The model under review builds one solid part; all positions refer to its coordinate system, in mm. A direction names the side the tool comes from. Coordinates: 2 decimals unless noted, no trailing zeros. Loops run counter-clockwise (first coordinate to the right, second up) from the corner with the lowest first, then second, coordinate; pieces in that order, holes last. Notation, with made-up numbers: M 42.25,77.25 L 59.25,77.25 A17 ccw 59.25,106.25 Z; hole C -4,35.5 d11. An arc over 180 degrees is marked long. Use one line per item in the form item = value.
```python
from build123d import *

# Parameters (mm, degrees)
F2_W = 0.2
F2_H = 0.2


with BuildPart() as f1:
    # F0 (on Right) → F1 (revolve)
    with BuildSketch(Plane.YZ):
        Polygon((-1.5, 0.5), (-1.5, 0), (9.2, 0), (9.2, 0.5), (7.7, 0.5), (7.7, 1.2), (6.2, 1.2), (6.2, 0.5), (3, 0.5), (3, 1.4), (0, 1.4), (0, 0.5), align=None)
    revolve(axis=Axis((0, 3.85, 0), (0, -1, 0)))

    # F2 (on Right) → F3 (revolve, cut)
    with BuildSketch(Plane.YZ):
        with Locations((0.1, 1.3)):
            Rectangle(F2_W, F2_H)
        with Locations((2.9, 1.3)):
            Rectangle(F2_W, F2_H)
    revolve(axis=Axis((0, 1.5, 0), (0, 1, 0)), mode=Mode.SUBTRACT)

    # F4 (on Right) → F5 (revolve)
    with BuildSketch(Plane.YZ):
        Polygon((6.3, 1.2), (6.7, 1.2), (7.6, 1.2), (7.6, 1.4), (6.3, 1.4), align=None)
    revolve(axis=Axis((0, 6.95, 0), (0, 1, 0)))


solid = f1.part
```
1. Add section D-D (y = 8). State the section outline as (x, z) points.
Response values:
outline = C 0,0 d1
2. Add section B-B (x = -0.65). State the section outline as (y, z) points, then the cut area to 3 significant figures.
Response values:
outline = M 0,-1.01 L 0.2,-1.01 L 0.2,-1.24 L 2.8,-1.24 L 2.8,-1.01 L 3,-1.01 L 3,1.01 L 2.8,1.01 L 2.8,1.24 L 0.2,1.24 L 0.2,1.01 L 0,1.01 Z; M 6.2,-1.01 L 6.3,-1.01 L 6.3,-1.24 L 7.6,-1.24 L 7.6,-1.01 L 7.7,-1.01 L 7.7,1.01 L 7.6,1.01 L 7.6,1.24 L 6.3,1.24 L 6.3,1.01 L 6.2,1.01 Z
area = 10.9 mm^2
3. The part is to be moulded in two halves that separate along Y. For faces 4 (the face through (0.488, 8.439, -0.108)), 5 (the face through (1, 3, 0)), 6 (the face through (1, 7.7, 0)), 7 (the face through (0, -1.5, 0)), say which applies: pulls with the +Y half, pulls with the -Y half, needs draft (parallel to the pull), parting line crosses it, or undercut.
Response values:
face_4 = needs draft
face_5 = undercut
face_6 = pulls with the +Y half
face_7 = pulls with the -Y half
4. Add section A-A (z = 0.65). State the section outline as (x, y) points, then the cut area to 3 significant figures.
Response values:
outline = M -1.24,0.2 L -1.01,0.2 L -1.01,0 L 1.01,0 L 1.01,0.2 L 1.24,0.2 L 1.24,2.8 L 1.01,2.8 L 1.01,3 L -1.01,3 L -1.01,2.8 L -1.24,2.8 Z; M -1.24,6.3 L -1.01,6.3 L -1.01,6.2 L 1.01,6.2 L 1.01,6.3 L 1.24,6.3 L 1.24,7.6 L 1.01,7.6 L 1.01,7.7 L -1.01,7.7 L -1.01,7.6 L -1.24,7.6 Z
area = 10.9 mm^2
5. Wall thickness on line 1 along Y through (x, z) = (-0.95, -0.65); line 2 along Y through (x, z) = (-1.1, 0.8); line 3 along X through (y, z) = (5, -0.15): over which ranges is each line inside the solid? List them lowest first. Write a range as from..to.
Response values:
line_1 = 0..3, 6.2..7.7
line_2 = 0.2..2.8, 6.3..7.6
line_3 = -0.48..0.48
6. Machinability: for faces 1 (the face through (1, 6.2, 0)), 2 (the face through (0.06, 6.94, -1.4)), 3 (the face through (1, 0, 0)), which of the approach directions +Z, -Z, +X, -X, +Y, -Y give a long, thin tool a straight path to every point of the face, cutting with its end or side? Answer none if there is none.
Response values:
face_1 = none
face_2 = +Y, -Y
face_3 = -Y
7. Add section C-C (y = 1). State the section outline as (x, z) points.
Response values:
outline = C 0,0 d2.8
